Autodesk Inventor part; units mm, degrees
ref_plane "YZ Plane" through (0, 0, 0) normal (1, 0, 0) x (0, 1, 0)
ref_plane "XZ Plane" through (0, 0, 0) normal (0, 1, 0) x (-1, 0, 0)
ref_plane "XY Plane" through (0, 0, 0) normal (0, 0, 1) x (1, 0, 0)
sketch "Náčrt1" plane through (0, 0, 0) normal (0, 1, 0) x (-1, 0, 0)
  line L0 (0, 0) -> (-30, 0)
  line L1 (-30, 0) -> (-30, -180)
  line L2 (-30, -180) -> (0, -180)
  line L3 (0, -180) -> (0, 0)
  dimension "d0" = 30
  dimension "d1" = 180
extrude "Vysunutí1" add sketch "Náčrt1" along normal blind 4
sketch "Náčrt2" plane through (0, 4, 0) normal (0, 1, 0) x (1, 0, 0)
  line L0 (30, 0) -> (30, 180)
  line L1 (30, 180) -> (0, 180)
  line L2 (0, 180) -> (0, 0)
  line L3 (0, 0) -> (30, 0)
  line L4 (15, 0) -> (15, 180) construction
  line L5 (9.65, 84.5) -> (20.35, 84.5)
  line L6 (20.35, 84.5) -> (20.35, 120)
  line L7 (20.35, 120) -> (9.65, 120)
  line L8 (9.65, 120) -> (9.65, 84.5)
  line L9 (12, 109.5) -> (18, 109.5)
  line L10 (18, 109.5) -> (18, 120)
  line L11 (18, 120) -> (12, 120)
  line L12 (12, 120) -> (12, 109.5)
  line L13 (18, 120) -> (20.35, 116.5)
  line L14 (12, 120) -> (9.65, 116.5)
  dimension "d4" = 10.7
  dimension "d5" = 35.5
  dimension "d6" = 60
  dimension "d7" = 6
  dimension "d8" = 10.5
  dimension "d9" = 32
extrude "Vysunutí2" cut sketch "Náčrt2" against normal blind 2 contours L8 L14 L12 L9 L10 L13 L6 L5
extrude "Vysunutí3" cut sketch "Náčrt2" against normal blind 4 contours L7 L10 L9 L12
sketch "Náčrt3" plane through (0, 4, 0) normal (0, 1, 0) x (1, 0, 0)
  circle A0 centre (15, 70) radius 4.75
  line L0 (30, 0) -> (30, 180)
  line L1 (30, 180) -> (0, 180)
  line L2 (0, 180) -> (0, 0)
  line L3 (0, 0) -> (30, 0)
  line L4 (12, 120) -> (18, 120)
  line L5 (18, 120) -> (20.35, 116.5)
  line L6 (20.35, 116.5) -> (20.35, 84.5)
  line L7 (20.35, 84.5) -> (9.65, 84.5)
  line L8 (9.65, 84.5) -> (9.65, 116.5)
  line L9 (9.65, 116.5) -> (12, 120)
  line L10 (15, 0) -> (15, 180) construction
  line L11 (12.3, 67.3) -> (17.7, 67.3)
  line L12 (17.7, 67.3) -> (17.7, 72.7)
  line L13 (17.7, 72.7) -> (12.3, 72.7)
  line L14 (12.3, 72.7) -> (12.3, 67.3)
  line L15 (0, 66.5) -> (30, 66.5)
  line L16 (30, 66.5) -> (30, 73.5)
  line L17 (30, 73.5) -> (0, 73.5)
  line L18 (0, 73.5) -> (0, 66.5)
  point P0 (11.7887, 73.5)
  point P1 (11.7887, 66.5)
  point P2 (18.2113, 73.5)
  point P3 (18.2113, 66.5)
  dimension "d14" = 9.5
  dimension "d15" = 70
  dimension "d16" = 5.4
  dimension "d17" = 5.4
  dimension "d18" = 2.7
  dimension "d19" = 7
  dimension "d20" = 3.5
extrude "Vysunutí4" cut sketch "Náčrt3" against normal blind 2 contours A0 L17 L0 L15 | A0 L15 L2 L17
extrude "Vysunutí5" cut sketch "Náčrt3" against normal blind 3 contours A0 L15 L17 | L17 A0 | A0 L15
extrude "Vysunutí6" cut sketch "Náčrt3" against normal blind 4 contours L14 L13 L12 L11
sketch "Náčrt4" plane through (0, 2, 0) normal (0, 1, 0) x (1, 0, 0)
  line L0 (20.35, 116.5) -> (20.35, 84.5) construction
  line L1 (18, 120) -> (20.35, 116.5) construction
  line L2 (18, 109.5) -> (18, 120) construction
  line L3 (12, 109.5) -> (18, 109.5) construction
  line L4 (12, 120) -> (12, 109.5) construction
  line L5 (9.65, 116.5) -> (12, 120) construction
  line L6 (9.65, 84.5) -> (9.65, 116.5) construction
  line L7 (20.35, 84.5) -> (9.65, 84.5) construction
  line L8 (9.65, 88.5) -> (20.35, 88.5)
  line L9 (20.35, 88.5) -> (20.35, 96.5)
  line L10 (20.35, 96.5) -> (9.65, 96.5)
  line L11 (9.65, 96.5) -> (9.65, 88.5)
  ellipse E0 centre (12.85, 98.5) end of major axis (14.1807, 98.5) minor radius 0.6195
  point P0 (0, 0)
  dimension "d27" = 8
  dimension "d28" = 4
  dimension "d29" = 14
  dimension "d30" = 3.2
extrude "Vysunutí7" cut sketch "Náčrt4" against normal blind 4 contours E0
extrude "Vysunutí8" cut sketch "Náčrt4" against normal blind 1 contours L11 L10 L9 L8
sketch "Náčrt5" plane through (0, 4, 0) normal (0, 1, 0) x (1, 0, 0)
  line L0 (0, 0) -> (30, 0)
  line L1 (0, 66.5) -> (0, 0)
  line L2 (15, 0) -> (15, 180) construction
  line L3 (30, 180) -> (0, 180) construction
  line L4 (30, 0) -> (30, 180) construction
  line L5 (30, 90) -> (0, 90) construction
  point P0 (3, 3)
  point P1 (27, 3)
  point P2 (3, 177)
  point P3 (27, 177)
  dimension "d35" = 3
  dimension "d36" = 3
hole "Díra1" at (3, 4, -3) at (27, 4, -3) at (3, 4, -177) at (27, 4, -177) direction (0, -1, 0) diameter 2 end through all
fillet "Zaoblení1" radius 1 4 edges at (27, 4, -4) (3, 4, -4) (27, 4, -178) (3, 4, -178)
equation "\"d20\" = 0.5 * d19"
properties part number "BackboardV3"
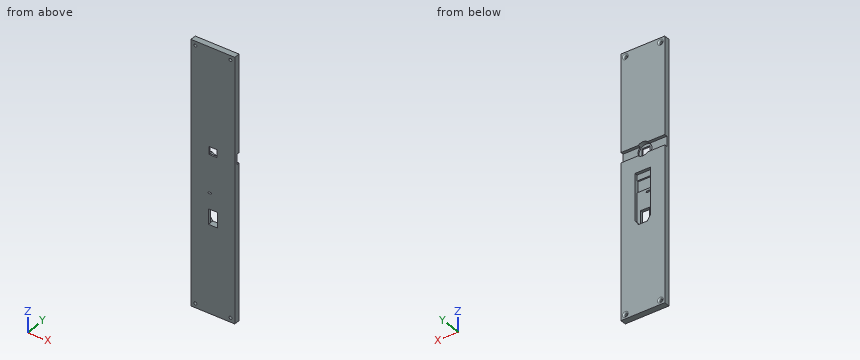
Part model, mm, in its own coordinate system. Round coordinates to 2 decimals unless told otherwise and drop trailing zeros. Loops run counter-clockwise (first coordinate to the right, second up) from the corner with the lowest first, then second, coordinate; pieces in that order, holes last.
1. Drill centre lines: line 1 along X through (y, z) = (1.75, -3); line 2 along Z through (x, y) = (5, 2.4); line 3 along Z through (x, y) = (13.5, 2.1). Where is each one in solid material? Low to high.
Solutions:
line 1: x = 0 to 2, 4 to 26, 28 to 30
line 2: z = -180 to -73.5, -66.5 to 0
line 3: z = -180 to -120, -84.5 to -74.51, -65.49 to 0
2. Slice it at A-A (z = -70). Give the cut face in (x, y), and give its area (3 significant figures).
Solutions:
outline: (0, 0) - (12.3, 0) - (12.3, 1) - (10.25, 1) - (10.25, 2) - (0, 2) - close; (17.7, 0) - (30, 0) - (30, 2) - (19.75, 2) - (19.75, 1) - (17.7, 1) - close
area: 45.1 mm2
3. Flat gauge pins, fed straight in: pin 1 (2 mm diameter, centred on x = 26, z = -70.5, fed in from +Y); pin 2 (1.2 mm diameter, centred on x = 3, z = -3, fed in from +Y). Where does each tip first touch, or does it go through?
Solutions:
pin 1: stops at y = 2
pin 2: passes through
